```python
from build123d import *

# Parameters (mm, degrees)
SKETCH_1_W             = 350
SKETCH_1_H             = 21
EXTRUDE_1_DEPTH        = 2
SKETCH_2_R             = 2
EXTRUDE_2_DEPTH        = 2
FILLET_1_R             = 10
SKETCH_3_R             = 1.5
CUT_EXTRUDE_1_DEPTH    = 30
PATTERN_LINEAR_1_COUNT = 10
PATTERN_LINEAR_1_PITCH = 30
SKETCH_4_R             = 1.5
CUT_EXTRUDE_2_DEPTH    = 10
CUT_EXTRUDE_3_DEPTH    = 5
PATTERN_LINEAR_2_COUNT = 11
PATTERN_LINEAR_2_PITCH = 30


with BuildPart() as part:
    # 草图1 → 凸台-拉伸1 (new body)
    with BuildSketch(Plane.XY):
        Rectangle(SKETCH_1_W, SKETCH_1_H)
    extrude(amount=EXTRUDE_1_DEPTH)

    # 草图2 → 凸台-拉伸2 (add)
    # profile 1 of 2: a face of its own
    with BuildSketch(Plane.XY.offset(2)):
        with BuildLine():
            Line((-175, -21), (-175, -10.5))
            Line((-175, -10.5), (-167, -10.5))
            Line((-167, -10.5), (-167, -21))
            ThreePointArc((-167, -21), (-171, -25), (-175, -21))
        make_face()
        with Locations((-171, -21)):
            Circle(SKETCH_2_R, mode=Mode.SUBTRACT)
    # profile 2 of 2: a face of its own
    with BuildSketch(Plane.XY.offset(2)):
        with BuildLine():
            Line((175, 20.5), (175, 10.5))
            Line((175, 10.5), (165, 10.5))
            Line((165, 10.5), (165, 20.5))
            ThreePointArc((165, 20.5), (170, 25.5), (175, 20.5))
        make_face()
        with Locations((170, 20.5)):
            Circle(SKETCH_2_R, mode=Mode.SUBTRACT)
    extrude(amount=-EXTRUDE_2_DEPTH)

    # 圆角1
    fillet_1_edges = [part.edges().sort_by_distance(p)[0] for p in [
        (-167, -10.5, 1),
        (165, 10.5, 1),
    ]]
    fillet(fillet_1_edges, radius=FILLET_1_R - 0.0001)  # a hair under: the kernel refuses the full size

    # 草图3 → 切除-拉伸1 (cut, symmetric)
    with BuildSketch(Plane.XY.offset(2)):
        with Locations((-137.5, 0)):
            Circle(SKETCH_3_R)
    cut_extrude_1 = extrude(amount=CUT_EXTRUDE_1_DEPTH, both=True, mode=Mode.SUBTRACT)

    # 阵列(线性)1: 切除-拉伸1 ×10
    with Locations(*[(i * PATTERN_LINEAR_1_PITCH, 0, 0) for i in range(1, PATTERN_LINEAR_1_COUNT)]):
        add(cut_extrude_1, mode=Mode.SUBTRACT)

    # 草图4 → 切除-拉伸2 (cut)
    with BuildSketch(Plane.XY.offset(2)):
        with Locations((-167.5, 0)):
            Circle(SKETCH_4_R)
        with Locations((162.5, 0)):
            Circle(SKETCH_4_R)
    extrude(amount=-CUT_EXTRUDE_2_DEPTH, mode=Mode.SUBTRACT)

    # 草图5 → 切除-拉伸3 (cut)
    with BuildSketch(Plane.XY.offset(2)):
        with BuildLine():
            Line((-157.5, 6), (-147.5, 6))
            ThreePointArc((-147.5, 6), (-141.5, 0), (-147.5, -6))
            Line((-147.5, -6), (-157.5, -6))
            ThreePointArc((-157.5, -6), (-163.5, 0), (-157.5, 6))
        make_face()
    cut_extrude_3 = extrude(amount=-CUT_EXTRUDE_3_DEPTH, mode=Mode.SUBTRACT)

    # 阵列(线性)2: 切除-拉伸3 ×11
    with Locations(*[(i * PATTERN_LINEAR_2_PITCH, 0, 0) for i in range(1, PATTERN_LINEAR_2_COUNT)]):
        add(cut_extrude_3, mode=Mode.SUBTRACT)


solid = part.part
```
Input: part model. Units: mm. Frame: model coordinates. A direction names the side the tool comes from. Coordinates: 2 decimals unless noted, no trailing zeros. Loops run counter-clockwise (first coordinate to the right, second up) from the corner with the lowest first, then second, coordinate; pieces in that order, holes last. Notation, with made-up numbers: M 8.25,29 L 12.25,29 A9 ccw 12.25,34 Z; hole C -2.75,45.25 d5. An arc over 180 degrees is marked long. One line per item, written item: value.
(1) Section A-A (x = 117). Output: boundary loops of the cut face in (y, z).
Filled in:
outline: M -10.5,0 L -6,0 L -6,2 L -10.5,2 Z; M 6,0 L 10.5,0 L 10.5,2 L 6,2 Z
(2) Reachability of faces 1 (the flat face through (1, 8, 2)), 2 (the cylindrical face through (158.5, 0.1, 1)) from +Z, -Z, +X, -X, +Y, -Y: full face, straight path, thin tool, end or side. Return the list, or none.
Filled in:
face 1: +Z, +X, -X, +Y, -Y
face 2: +Z, -Z
(3) Line query: line 1 along Y through (x, z) = (-47.5, 1.65); line 2 along Y through (x, z) = (-167.5, 1.6); line 3 along Y through (x, z) = (-50, 1.35). Output: solid intervals per line, ascending. Write a range as from..to.
Filled in:
line 1: -10.5..-1.5, 1.5..10.5
line 2: -22.94..-1.5, 1.5..10.5
line 3: -10.5..10.5
(4) Pin query (flat end, axial travel): pin 1 (1 mm diameter, centred on x = -154.5, z = 1, fed in from +Y); pin 2 (1 mm diameter, centred on x = -64, z = 0.5, fed in from -Y). Return the tip coordinate at first contact, or that it passes through.
Filled in:
pin 1: y = 10.5
pin 2: y = -10.5
(5) Section B-B (z = 1.3). Give the number of separate pieces and of enclosed holes in the cut face, and give its area (3 significant figures).
Filled in:
separate pieces: 1
enclosed holes: 25
area: 4,970 mm^2
(6) Pull-direction query (X, two-part tool) for faces 3 (the flat face through (1, 8, 0)), 4 (the cylindrical face through (-164.15, -13.51, 0.99)), 5 (the cylindrical face through (162.15, 13.51, 0.99)), 6 (the cylindrical face through (-13.5, -0.1, 1)); classes: +X half, -X half, draft (parallel to the pull), parting line (faces both ways), or undercut.
Filled in:
face 3: draft
face 4: +X half
face 5: -X half
face 6: undercut
